Verification items for the finished model (mm, model axes). A direction names the side the tool comes from. Give positions to 0.01 mm unless a question says otherwise; leave off trailing zeros. Order: outer loops, then holes, each group sorted by start corner. A loop starts at its lowest first (then second) coordinate and runs counter-clockwise, first axis right, second up. Notation, with made-up numbers: (-8.5, -21) - (31.5, -21) arc R25 cw to (31.5, -8) - close; hole circle Ø6 at (74.5, -38). An arc over 180 degrees is marked (long way). Answer as a JSON object with one key per item and string values.
Solid Edge part; units mm, degrees
sketch "Sketch1" plane through (0, 0, 0) normal (0, -1, 0) x (1, 0, 0)
  line L0 (-1.9, 29.8) -> (-1.9, -29.8)
  arc A0 (-1.9, -29.8) -> (-6.9, -34.8) centre (-6.9, -29.8) cw
  line L1 (-23, -34.8) -> (-6.9, -34.8)
  line L2 (-23, -40) -> (-23, -34.8)
  line L3 (23, -40) -> (-23, -40)
  line L4 (23, -40) -> (23, -34.8)
  line L5 (23, -34.8) -> (6.9, -34.8)
  arc A1 (1.9, -29.8) -> (6.9, -34.8) centre (6.9, -29.8) ccw
  line L6 (1.9, -29.8) -> (1.9, 29.8)
  arc A2 (6.9, 34.8) -> (1.9, 29.8) centre (6.9, 29.8) ccw
  line L7 (23, 34.8) -> (6.9, 34.8)
  line L8 (23, 40) -> (23, 34.8)
  line L9 (-23, 40) -> (23, 40)
  line L10 (-23, 34.8) -> (-23, 40)
  line L11 (-23, 34.8) -> (-6.9, 34.8)
  arc A3 (-6.9, 34.8) -> (-1.9, 29.8) centre (-6.9, 29.8) cw
  dimension "D1" = 23
  dimension "D2" = 23
extrude "Protrusion1" add sketch "Sketch1" against normal blind 25.4
(1) Section check C-C (z = 18). Record the cut outline in (x, y).
Computed values:
{"outline": "(-1.9, 0) - (1.9, 0) - (1.9, 25.4) - (-1.9, 25.4) - close"}
(2) Gauge pin test, flat ends, axial feed: pin 1 Ø12.5 at (y, z) = (11.5, 1.5) entering from -X; pin 2 Ø6 at (x, z) = (-3, -30.5) entering from +Y; pin 3 Ø8 at (x, z) = (-9, 15) entering from +Y. Record the tip position at first contact, or that the pin passes through.
Computed values:
{"pin 1": "stops at x = -1.9", "pin 2": "stops at y = 25.4", "pin 3": "passes through"}
(3) Release check for a two-part mould opening along Z. For faces 1 (the flat face through (0, 25.4, 0)), 2 (the cylindrical face through (3.4, 12.52, 33.37)), 3 (the flat face through (0, 13, -40)) record: pulls with the +Z half, pulls with the -Z half, needs draft (parallel to the pull), parting line crosses it, or undercut.
Computed values:
{"face 1": "needs draft", "face 2": "undercut", "face 3": "pulls with the -Z half"}
(4) Material ranges on line 1 along Z through (x, y) = (13, 9.75); line 2 along X through (y, z) = (7.5, -7.5); line 3 along Z through (x, y) = (5, 2.5), recorded low to high. Write a range as [from, to].
Computed values:
{"line 1": "z = [-40, -34.8], [34.8, 40]", "line 2": "x = [-1.9, 1.9]", "line 3": "z = [-40, -34.42], [34.42, 40]"}
(5) Section check B-B (y = 21.25). Record the cut outline in (x, z).
Computed values:
{"outline": "(-23, -40) - (23, -40) - (23, -34.8) - (6.9, -34.8) arc R5 cw to (1.9, -29.8) - (1.9, 29.8) arc R5 cw to (6.9, 34.8) - (23, 34.8) - (23, 40) - (-23, 40) - (-23, 34.8) - (-6.9, 34.8) arc R5 cw to (-1.9, 29.8) - (-1.9, -29.8) arc R5 cw to (-6.9, -34.8) - (-23, -34.8) - close"}
(6) Access from +Z, -Z, +X, -X, +Y, -Y to the whole of each face (thin tool, end or side, straight path). Record for faces 4 (the flat face through (-23, 13, -37)), 5 (the flat face through (15, 13, 34.8)), 6 (the flat face through (-15, 13, -34.8)).
Computed values:
{"face 4": "+Z, -Z, -X, +Y, -Y", "face 5": "+X, +Y, -Y", "face 6": "-X, +Y, -Y"}
(7) Section check A-A (x = 10.5). Record the cut outline in (y, z), then the cut area to 3 significant figures.
Computed values:
{"outline": "(0, -40) - (25.4, -40) - (25.4, -34.8) - (0, -34.8) - close; (0, 34.8) - (25.4, 34.8) - (25.4, 40) - (0, 40) - close", "area": "264 mm²"}
